Build history of the part. All positions in model axes, mm. A direction names the side the tool comes from. Give positions to 0.01 mm unless a question says otherwise; leave off trailing zeros. Order: outer loops, then holes, each group sorted by start corner. A loop starts at its lowest first (then second) coordinate and runs counter-clockwise, first axis right, second up. Notation, with made-up numbers: (52, 27.5) -> (59, 27.5) arc R20 ccw to (59, 56.5) -> close; hole circle Ø9 at (28, -15.75). An arc over 180 degrees is marked (long way). One line per question, with ' | ' between items. Start each with the question number.
(1) Cut at C-C (y = -16.5). Give the cut face in (x, z), then the cut area to 3 significant figures.
(2) Cut at A-A (z = 3.5). Give the cut face in (x, y), then the cut area to 3 significant figures.
(3) Pull direction Y, two halves, no side cores. Call faces 4 (the face through (-60.706, -26, 4)), 5 (the face through (64, -22.606, 4)), 6 (the face through (-58.166, 23, 4)), 7 (the face through (-1, 28.956, 4)): +Y half, -Y half, draft (parallel to the pull), parting line (faces both ways), or undercut.
(4) Drill centre lines: L1, parallel to X at y = 26, z = 1.35; L2, parallel to X at y = -5, z = 4.25; L3, parallel to Y at x = 20, z = 4.3. Where is each one in solid material? Low to high. Write a range as from..to.
(5) Which spindle directions (+Z, -Z, +X, -X, +Y, -Y) get a long thin tool onto all of the face, cutting with end or side? Do faces 1 (the face through (-61, -20.066, 4)), 2 (the face through (60.706, -26, 4)), 3 (the face through (-64, -22.606, 4)). Say none if no direction does.
(6) Pin check, flat tips, straight feed: pin 1 Ø2 at (y, z) = (-23, 4.5) entering from +X; pin 2 Ø6 at (x, y) = (45, -18.5) entering from +Z; pin 3 Ø1.3 at (y, z) = (26.5, 3.5) entering from -X; pin 4 Ø1.4 at (x, y) = (-64.135, 26.035) entering from -Z. Stop position of each tip, or through.
(7) Cut at B-B (x = 43). Give the cut face in (y, z), then the cut area to 3 significant figures.
from build123d import *

# Parameters (mm, degrees)
F0_W     = 139.7
F0_H     = 63.5
F1_DEPTH = 2.54
F2_W     = 134.112
F2_H     = 57.912
F3_DEPTH = 2.54
F4_W     = 6.35
F4_H     = 6.35
F5_DEPTH = 2.54
F7_DEPTH = 2.54
F8_R     = 1.143
F9_DEPTH = 2.54


with BuildPart() as f1:
    # F0 (on Top) → F1 (new body)
    with BuildSketch(Plane.XY):
        Rectangle(F0_W, F0_H)
    extrude(amount=F1_DEPTH)

    # F2 (on face) → F3 (join)
    with BuildSketch(Plane.XY.offset(2.54)):
        Rectangle(F2_W, F2_H)
    extrude(amount=F3_DEPTH)

    # F4 (on face) → F5 (cut)
    with BuildSketch(Plane.XY.offset(5.08)):
        with Locations((-63.881, 25.781)):
            Rectangle(F4_W, F4_H)
        with Locations((63.881, 25.781)):
            Rectangle(F4_W, F4_H)
        with Locations((-63.881, -25.781)):
            Rectangle(F4_W, F4_H)
        with Locations((63.881, -25.781)):
            Rectangle(F4_W, F4_H)
    extrude(amount=-F5_DEPTH, mode=Mode.SUBTRACT)

    # F6 (on face) → F7 (cut)
    with BuildSketch(Plane.XY.offset(5.08)):
        Polygon((64.516, 20.066), (58.166, 20.066), (58.166, 26.416), (-58.166, 26.416), (-58.166, 20.066), (-64.516, 20.066), (-64.516, -20.066), (-58.166, -20.066), (-58.166, -26.416), (58.166, -26.416), (58.166, -20.066), (64.516, -20.066), align=None)
    extrude(amount=-F7_DEPTH, mode=Mode.SUBTRACT)

    # F8 (on face) → F9 (cut, through all)
    with BuildSketch(Plane(origin=(0, 0, 0), x_dir=(1, 0, 0), z_dir=(0, 0, -1))):
        with Locations((64.135, 26.035)):
            Circle(F8_R)
        with Locations((-64.135, 26.035)):
            Circle(F8_R)
        with Locations((64.135, -26.035)):
            Circle(F8_R)
        with Locations((-64.135, -26.035)):
            Circle(F8_R)
    extrude(amount=-F9_DEPTH, mode=Mode.SUBTRACT)


solid = f1.part
Result set:
1) outline: (-69.85, 0) -> (69.85, 0) -> (69.85, 2.54) -> (67.06, 2.54) -> (67.06, 5.08) -> (64.52, 5.08) -> (64.52, 2.54) -> (-64.52, 2.54) -> (-64.52, 5.08) -> (-67.06, 5.08) -> (-67.06, 2.54) -> (-69.85, 2.54) -> close | area: 368 mm2
2) outline: (-67.06, -22.61) -> (-60.71, -22.61) -> (-60.71, -28.96) -> (60.71, -28.96) -> (60.71, -22.61) -> (67.06, -22.61) -> (67.06, 22.61) -> (60.71, 22.61) -> (60.71, 28.96) -> (-60.71, 28.96) -> (-60.71, 22.61) -> (-67.06, 22.61) -> close; hole (-64.52, -20.07) -> (-58.17, -20.07) -> (-58.17, -26.42) -> (58.17, -26.42) -> (58.17, -20.07) -> (64.52, -20.07) -> (64.52, 20.07) -> (58.17, 20.07) -> (58.17, 26.42) -> (-58.17, 26.42) -> (-58.17, 20.07) -> (-64.52, 20.07) -> close | area: 950 mm2
3) face 4: draft | face 5: -Y half | face 6: undercut | face 7: +Y half
4) L1: x = -69.85..-65.28, -62.99..62.99, 65.28..69.85 | L2: x = -67.06..-64.52, 64.52..67.06 | L3: y = -28.96..-26.42, 26.42..28.96
5) face 1: +Z | face 2: +Z, +X, -Y | face 3: +Z, -X, -Y
6) pin 1: stops at x = 67.06 | pin 2: stops at z = 2.54 | pin 3: stops at x = -60.71 | pin 4: passes through
7) outline: (-31.75, 0) -> (31.75, 0) -> (31.75, 2.54) -> (28.96, 2.54) -> (28.96, 5.08) -> (26.42, 5.08) -> (26.42, 2.54) -> (-26.42, 2.54) -> (-26.42, 5.08) -> (-28.96, 5.08) -> (-28.96, 2.54) -> (-31.75, 2.54) -> close | area: 174 mm2
